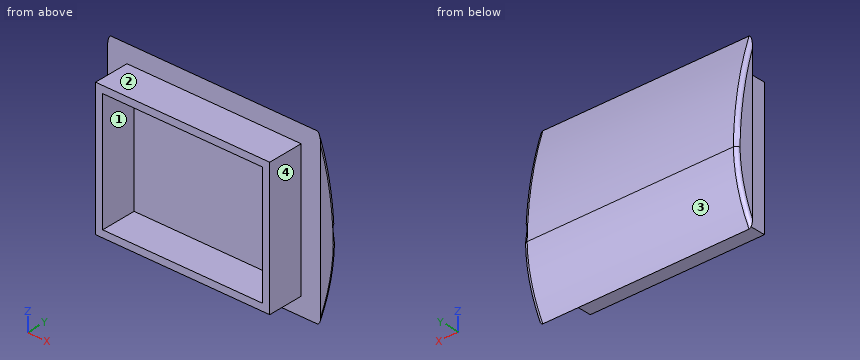
from build123d import *

# Parameters (mm, degrees)
SKETCH1_W                = 124.46
SKETCH1_H                = 95.504
BOSS_EXTRUDE1_DEPTH      = 25.4
BOSS_EXTRUDE2_DEPTH      = 76.2
BOSS_EXTRUDE2_DEPTH_BACK = 76.2
SKETCH4_W                = 114.3
SKETCH4_H                = 85.344
CUT_EXTRUDE1_DEPTH       = 25.4
FILLET3_R                = 2.54


with BuildPart() as part:
    # Sketch1 → Boss-Extrude1 (new body)
    with BuildSketch(Plane(origin=(0, 0, 0), x_dir=(1, 0, 0), z_dir=(0, 1, 0))):
        with Locations((0, -3.048)):
            Rectangle(SKETCH1_W, SKETCH1_H)
    extrude(amount=BOSS_EXTRUDE1_DEPTH)

    # Sketch3 → Boss-Extrude2 (add, two sides: drawn at the far end of the back side and taken through both)
    with BuildSketch(Plane(origin=(0, 0, 0), x_dir=(0, 0, -1), z_dir=(1, 0, 0)).offset(-BOSS_EXTRUDE2_DEPTH_BACK)):
        with BuildLine():
            ThreePointArc((11.684, 38.1), (35.337321444, 34.605957197), (57.404, 25.4))
            Line((57.404, 25.4), (44.704, 25.4))
            Line((44.704, 25.4), (11.684, 25.4))
            Line((11.684, 25.4), (11.684, 38.1))
        make_face()
        with BuildLine():
            ThreePointArc((-63.5, 25.4), (-26.387271572, 34.587287709), (11.684, 38.1))
            Line((11.684, 38.1), (11.684, 25.4))
            Line((11.684, 25.4), (-50.8, 25.4))
            Line((-50.8, 25.4), (-63.5, 25.4))
        make_face()
    extrude(amount=BOSS_EXTRUDE2_DEPTH + BOSS_EXTRUDE2_DEPTH_BACK)

    # Sketch4 → Cut-Extrude1 (cut)
    with BuildSketch(Plane.XZ):
        with Locations((0, 3.048)):
            Rectangle(SKETCH4_W, SKETCH4_H)
    extrude(amount=-CUT_EXTRUDE1_DEPTH, mode=Mode.SUBTRACT)

    # Fillet3
    fillet3_edges = [part.edges().sort_by_distance(p)[0] for p in [
        (76.2, 34.605957197, -35.337321444),
        (76.2, 34.587287709, 26.387271572),
        (-76.2, 34.605957197, -35.337321444),
        (-76.2, 34.587287709, 26.387271572),
    ]]
    fillet(fillet3_edges, radius=FILLET3_R)


solid = part.part
Geometry check sheet. Reference: the model listing, model coordinates, mm. Face numbers are marked on the shaded views. A direction names the side the tool comes from. Coordinates: 2 decimals unless noted, no trailing zeros. Order: outer loops, then holes, each group sorted by start corner. A loop starts at its lowest first (then second) coordinate and runs counter-clockwise, first axis right, second up. Notation, with made-up numbers: (53.25, 56) - (85.25, 56) arc R16 cw to (85.25, 82) - close; hole circle Ø3 at (6.5, 0.25). An arc over 180 degrees is marked (long way). One line per item, written item: value.
(1) Access from +Z, -Z, +X, -X, +Y, -Y to the whole of each face (thin tool, end or side, straight path). Record for the marked faces 1, 2, 3 and 4.
Data:
face 1: -Y
face 2: +Z, +X, -X, -Y
face 3: -Z, +X, -X, +Y
face 4: +Z, -Z, +X, -Y
(2) Sectioned sample at A-A (y = 19). Enter the section's corners in (x, z).
Data:
outline: (-62.23, -44.7) - (62.23, -44.7) - (62.23, 50.8) - (-62.23, 50.8) - close; hole (-57.15, -39.62) - (57.15, -39.62) - (57.15, 45.72) - (-57.15, 45.72) - close
(3) Thickness scan on probe 1 along X at (y, z) = (11, 6); probe 2 along Z at (x, y) = (38, 14); probe 3 along Y at (x, z) = (-54, -12.5). Record the ranges inside material, lowest first. Write a range as from..to.
Data:
probe 1: x = -62.23..-57.15, 57.15..62.23
probe 2: z = -44.7..-39.62, 45.72..50.8
probe 3: y = 25.4..38.08
(4) Sectioned sample at B-B (x = 14.5). Enter the section's corners in (y, z).
Data:
outline: (0, -44.7) - (25.4, -44.7) - (25.4, -57.4) arc R96.44 ccw to (38.1, -11.68) arc R254 ccw to (25.4, 63.5) - (25.4, 50.8) - (0, 50.8) - (0, 45.72) - (25.4, 45.72) - (25.4, -39.62) - (0, -39.62) - close
(5) Depth check by flat-ended pin: pin 1 Ø8 at (x, z) = (-59, 35) entering from +Y; pin 2 Ø7.5 at (x, y) = (-19, 18) entering from +Z; pin 3 Ø1 at (y, z) = (15, 23.5) entering from -X; pin 4 Ø20.5 at (y, z) = (18.5, -1.5) entering from -X. Enter the tip coordinate at first touch or a pass-through.
Data:
pin 1: stops at y = 33.76
pin 2: stops at z = 50.8
pin 3: stops at x = -62.23
pin 4: stops at x = -76.2
